Autodesk Inventor part; units mm, degrees
ref_plane "YZ Plane" through (0, 0, 0) normal (1, 0, 0) x (0, 1, 0)
ref_plane "XZ Plane" through (0, 0, 0) normal (0, 1, 0) x (-1, 0, 0)
ref_plane "XY Plane" through (0, 0, 0) normal (0, 0, 1) x (1, 0, 0)
sketch "Sketch1" plane through (0, 0, 0) normal (1, 0, 0) x (0, 1, 0)
  line L0 (0, 0) -> (25.4, 0)
  line L1 (0, 0) -> (0, 75.184)
  line L2 (0, 75.184) -> (25.4, 0)
  dimension "d0" = 25.4
  dimension "d1" = 75.184
extrude "Extrusion1" add sketch "Sketch1" along normal blind 114.3
sketch "Sketch2" plane through (0, 0, 75.184) normal (0, 0.9473953, 0.320066) x (1, 0, 0)
  circle A0 centre (30.1625, 17.4625) radius 13.4874
  point P0 (0, 71.229)
  dimension "d4" = 26.9748
extrude "Extrusion2" add sketch "Sketch2" along normal blind 25.4
sketch "Sketch3" plane through (30.1625, 29.653, 66.7698) normal (0, 0.9473953, 0.320066) x (1, 0, 0)
  circle A0 centre (0, 0) radius 14.9075
  point P0 (-30.1625, 53.7665)
extrude "Extrusion3" cut sketch "Sketch3" against normal blind 76.2
sketch "Sketch4" plane through (0, 0, 0) normal (0, -1, 0) x (1, 0, 0)
  point P0 (0, 0)
sketch "Sketch5" plane through (0, 0, 0) normal (0, -1, 0) x (1, 0, 0)
  arc A0 (42.3045, 45.008) -> (44.45, 66.675) centre (30.1625, 57.15) ccw
  arc A1 (44.3808, 43.1924) -> (47.2504, 67.396) centre (30.1625, 57.15) ccw
  arc A2 (15.875, 66.675) -> (17.0779, 46.0302) centre (30.1625, 57.15) ccw
  arc A3 (13.625, 68.2625) -> (14.8563, 44.3948) centre (30.1625, 57.15) ccw
  line L0 (13.625, 68.2625) -> (15.875, 66.675)
  line L1 (14.8563, 44.3948) -> (17.0779, 46.0302)
  line L2 (44.45, 66.675) -> (47.2504, 67.396)
  line L3 (42.3045, 45.008) -> (44.3808, 43.1924)
  point P0 (0, 0)
extrude "Extrusion4" add sketch "Sketch5" along normal blind 5.08
sketch "Sketch6" plane through (0, 0, 75.184) normal (0, 0.9473953, 0.320066) x (1, 0, 0)
  line L0 (0, 79.3586) -> (114.3, 79.3586)
  line L1 (14.2875, 31.75) -> (11.1125, 31.75)
  line L2 (11.1125, 31.75) -> (11.1125, 79.3586)
  line L3 (11.1125, 79.3586) -> (14.2875, 79.3586)
  line L4 (14.2875, 79.3586) -> (14.2875, 31.75)
  line L5 (49.2743, 31.75) -> (45.5103, 31.75)
  line L6 (45.5103, 31.75) -> (45.5103, 79.375)
  line L7 (45.5103, 79.375) -> (49.2743, 79.375)
  line L8 (49.2743, 79.375) -> (49.2743, 31.75)
  point P0 (0, 71.229)
extrude "Extrusion5" add sketch "Sketch6" along normal blind 25.4
properties part number "CAP PROCESS SKETCH"
Build history of the part. All positions in model axes, mm. A direction names the side the tool comes from. Give positions to 0.01 mm unless a question says otherwise; leave off trailing zeros. Loops run counter-clockwise (first coordinate to the right, second up) from the corner with the lowest first, then second, coordinate; pieces in that order, holes last. Notation, with made-up numbers: (86.5, 60) -> (99.5, 60) arc R21 cw to (99.5, 78) -> close; hole circle Ø1 at (-19, -14.75). An arc over 180 degrees is marked (long way). One line per question, with ' | ' between items. Start each with the question number.
1) Cut at C-C (z = 19). Give the cut face in (x, y), plus the area to 3 significant figures.
2) Cut at D-D (y = 22). Give the cut face in (x, z).
3) Pin check, flat tips, straight feed: pin 1 (1.5 mm diameter, centred on x = 30, y = 4.5, fed in from +Z); pin 2 (22.5 mm diameter, centred on x = 76, z = 43, fed in from -Y); pin 3 (6 mm diameter, centred on y = 21.5, z = 42, fed in from +X). Stop position of each tip, or through.
4) Probe L1, parallel to X at y = 25, z = 40; L2, parallel to Y at x = 16, z = 33.5; L3, parallel to Y at x = 78.5, z = 22.5. List the from-to ranges inside material, lowest first.
5) Cut at B-B (y = 32). Give the cut face in (x, z).
6) 3-axis set-ups, long thin cutter, end or side, ignore diameter. For faces 1 (the flat face through (14.734, -2.504, 67.48)), 2 (the flat face through (12.722, 22.026, 49.112)), 3 (the flat face through (15.95, -2.5, 45.2)), 4 (the cylindrical face through (49.97, -2.5, 54.99)): which of +Z, -Z, +X, -X, +Y, -Y reach the whole face in a straight line?
7) Two-plate mould, pull along Z, no slides. Class faces 5 (the flat face through (56.35, 12.52, 38.12)), 6 (the flat face through (12.678, 37.263, 4.008)), 7 (the cylindrical face through (47.266, -2.504, 55.622)), 8 (the cylindrical face through (13.03, -2.5, 56)): released by +Z, released by -Z, zero draft, split by the parting line, or undercut.
8) Cut at A-A (x = 31.5). Give the cut face in (y, z).
Return value:
1) outline: (0, 0) -> (114.3, 0) -> (114.3, 18.98) -> (49.27, 18.98) -> (49.27, 45.79) -> (45.51, 45.79) -> (45.51, 18.98) -> (14.29, 18.98) -> (14.29, 45.79) -> (11.11, 45.79) -> (11.11, 18.98) -> (0, 18.98) -> close | area: 2,360 mm^2
2) outline: (0, 0) -> (114.3, 0) -> (114.3, 10.06) -> (49.27, 10.06) -> (49.27, 49.1) -> (45.51, 49.1) -> (45.51, 10.06) -> (14.29, 10.06) -> (14.29, 49.1) -> (11.11, 49.1) -> (11.11, 10.06) -> (0, 10.06) -> close
3) pin 1: z = 42.79 | pin 2: y = 0 | pin 3: x = 49.27
4) L1: 11.11 to 14.29, 45.51 to 49.27 | L2: 0 to 14.08 | L3: 0 to 17.8
5) outline: (11.11, 2.23) -> (14.29, 2.23) -> (14.29, 52.48) -> (11.11, 52.48) -> close; (45.51, 2.21) -> (49.27, 2.21) -> (49.27, 52.48) -> (45.51, 52.48) -> close
6) face 1: +Z, -Y | face 2: +Z, +X, -X | face 3: -Z, -Y | face 4: +X, -Y
7) face 5: released by +Z | face 6: released by -Z | face 7: undercut | face 8: undercut
8) outline: (0, 0) -> (25.4, 0) -> (10.34, 44.57) -> (0, 41.08) -> close; (0, 72.42) -> (0.84, 72.71) -> (0, 75.18) -> close
